Here's how the part is built. I have some questions about the finished solid (model axes, mm). Face numbers are marked on the shaded views. A direction names the side the tool comes from. Give positions to 0.01 mm unless a question says otherwise; leave off trailing zeros. Order: outer loops, then holes, each group sorted by start corner. A loop starts at its lowest first (then second) coordinate and runs counter-clockwise, first axis right, second up. Notation, with made-up numbers: (59, 46.25) -> (100, 46.25) arc R20 cw to (100, 53.25) -> close; hole circle Ø4 at (66, 23.5). An arc over 180 degrees is marked (long way). Write each question's results on one line, items separated by ' | '. Start each with the question number.
Q1. For the marked faces 3 and 4, which set-ups out of +Z, -Z, +X, -X, +Y, -Y let a thin tool reach every point of the face, with its end or its side?
Q2. Imagine slicing it at C-C, the plane y = -0.5. Please give me the cut outline in (x, z).
Q3. Imagine slicing it at D-D, the plane y = -2.75. Please give me the cut outline in (x, z), then the cut area to 3 significant figures.
Q4. Imagine slicing it at B-B, the plane x = 39.5. Please give me the cut outline in (y, z), then the cut area to 3 significant figures.
Q5. I'm going to push flat-ended pins straight in: pin 1 (4 mm diameter, centred on y = -2, z = 9.5, fed in from -X); pin 2 (1.2 mm diameter, centred on x = 0, z = 5.5, fed in from +Y); pin 3 (3 mm diameter, centred on x = -1, z = 7, fed in from -Y). Where does each tip first touch, or does it pass through?
Q6. I need wall thicknesses on line 1 along Z through (x, y) = (31, -2.75); line 2 along Y through (x, z) = (6, 1.5); line 3 along X through (y, z) = (0, 4.75). Which ranges of each line are inside material? Lowest first, please. Write a range as [from, to].
Q7. Imagine slicing it at A-A, the plane z = 4.75. Please give me the cut outline in (x, y), then the cut area to 3 significant figures.
Q8. Thinking about a two-plate mould opening in X: for the marked faces 1 and 2, which applies, pulls with the +X half, pulls with the -X half, needs draft (parallel to the pull), parting line crosses it, or undercut?
```python
from build123d import *

# Parameters (mm, degrees)
F1_DEPTH = 2
F2_DEPTH = 12
F3_DEPTH = 12


with BuildPart() as f1:
    # F0 (on Top) → F1 (new body)
    with BuildSketch(Plane.XY):
        with BuildLine():
            Line((3.5, 3.5), (3.5, 0))
            Line((3.5, 0), (5, 0))
            Line((5, 0), (5, 1.5))
            Line((5, 1.5), (45, 1.5))
            Line((45, 1.5), (45, 0))
            Line((45, 0), (46.5, 0))
            ThreePointArc((46.5, 0), (47.525126, 2.474874), (50, 3.5))
            Line((50, 3.5), (3.5, 3.5))
        make_face()
        with BuildLine():
            Line((5, 0), (3.5, 0))
            Line((3.5, 0), (3.5, -3.5))
            Line((3.5, -3.5), (50, -3.5))
            ThreePointArc((50, -3.5), (47.525126, -2.474874), (46.5, 0))
            Line((46.5, 0), (45, 0))
            Line((45, 0), (45, -1.5))
            Line((45, -1.5), (5, -1.5))
            Line((5, -1.5), (5, 0))
        make_face()
        Polygon((3.5, -3.5), (3.5, 0), (3.5, 3.5), (0, 3.5), (-3.5, 3.5), (-3.5, -3.5), (0, -3.5), align=None)
        Polygon((2, 1.25), (2, 0), (2, -1.25), (-2, -1.25), (-2, 1.25), align=None, mode=Mode.SUBTRACT)
        Polygon((2, -1.25), (2, 0), (2, 1.25), (-2, 1.25), (-2, -1.25), align=None)
        with BuildLine():
            ThreePointArc((46.5, 0), (47.525126, -2.474874), (50, -3.5))
            ThreePointArc((50, -3.5), (52.474874, -2.474874), (53.5, 0))
            ThreePointArc((53.5, 0), (52.474874, 2.474874), (50, 3.5))
            ThreePointArc((50, 3.5), (47.525126, 2.474874), (46.5, 0))
        make_face()
        with BuildLine():
            ThreePointArc((51.5, 0), (50, -1.5), (48.5, 0))
            ThreePointArc((48.5, 0), (50, 1.5), (51.5, 0))
        make_face(mode=Mode.SUBTRACT)
        with BuildLine():
            ThreePointArc((51.5, 0), (50, 1.5), (48.5, 0))
            ThreePointArc((48.5, 0), (50, -1.5), (51.5, 0))
        make_face()
    extrude(amount=F1_DEPTH)

    # F0 (on Top) → F2 (join)
    with BuildSketch(Plane.XY):
        Polygon((2, -1.25), (2, 0), (2, 1.25), (-2, 1.25), (-2, -1.25), align=None)
    extrude(amount=F2_DEPTH)

    # F0 (on Top) → F3 (join)
    with BuildSketch(Plane.XY):
        with BuildLine():
            ThreePointArc((51.5, 0), (50, 1.5), (48.5, 0))
            ThreePointArc((48.5, 0), (50, -1.5), (51.5, 0))
        make_face()
    extrude(amount=F3_DEPTH)


solid = f1.part
```
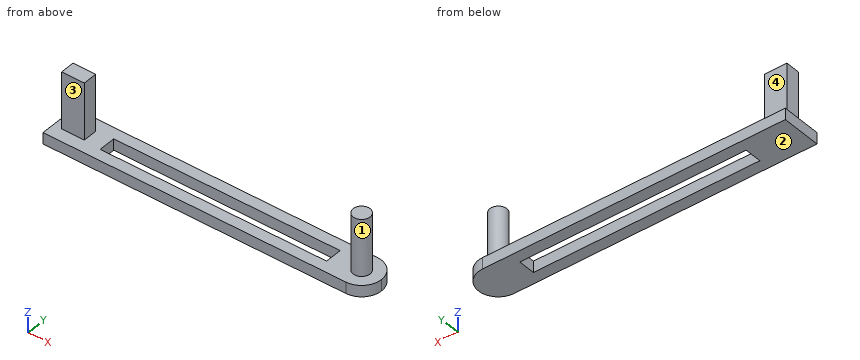
Geometry check:
1) face 3: +Z, -X, -Y | face 4: +Z, -X, +Y
2) outline: (-3.5, 0) -> (5, 0) -> (5, 2) -> (2, 2) -> (2, 12) -> (-2, 12) -> (-2, 2) -> (-3.5, 2) -> close; (45, 0) -> (53.46, 0) -> (53.46, 2) -> (51.41, 2) -> (51.41, 12) -> (48.59, 12) -> (48.59, 2) -> (45, 2) -> close
3) outline: (-3.5, 0) -> (52.17, 0) -> (52.17, 2) -> (-3.5, 2) -> close | area: 111 mm²
4) outline: (-3.5, 0) -> (-1.5, 0) -> (-1.5, 2) -> (-3.5, 2) -> close; (1.5, 0) -> (3.5, 0) -> (3.5, 2) -> (1.5, 2) -> close | area: 8.00 mm²
5) pin 1: x = -2 | pin 2: y = 1.25 | pin 3: y = -1.25
6) line 1: [0, 2] | line 2: [-3.5, -1.5], [1.5, 3.5] | line 3: [-2, 2], [48.5, 51.5]
7) outline: (-2, -1.25) -> (2, -1.25) -> (2, 1.25) -> (-2, 1.25) -> close; circle Ø3 at (50, 0) | area: 17.1 mm²
8) face 1: undercut | face 2: needs draft
